Autodesk Inventor part; units mm, degrees
ref_plane "YZ Plane" through (0, 0, 0) normal (1, 0, 0) x (0, 1, 0)
ref_plane "XZ Plane" through (0, 0, 0) normal (0, 1, 0) x (-1, 0, 0)
ref_plane "XY Plane" through (0, 0, 0) normal (0, 0, 1) x (1, 0, 0)
sketch "Sketch1" plane through (0, 0, 0) normal (0, 1, 0) x (-1, 0, 0)
  line L0 (-175, 200) -> (175, 200)
  line L1 (175, 200) -> (175, -200)
  line L2 (175, -200) -> (-175, -200)
  line L3 (-175, -200) -> (-175, 200)
  line L4 (-175, 200) -> (175, -200) construction
  line L5 (175, 200) -> (-175, -200) construction
  point P0 (0, 0)
  point P1 (0, 0)
  dimension "d0" = 350
  dimension "d1" = 400
extrude "Extrusion1" add sketch "Sketch1" along normal blind 2
sketch "Sketch2" plane through (0, 0, 0) normal (0, -1, 0) x (1, 0, 0)
  line L0 (175, 200) -> (175, -200) construction
  line L1 (-175, 200) -> (175, 200) construction
  line L2 (175, 155) -> (125, 155)
  line L3 (125, 155) -> (125, 135)
  line L4 (125, 135) -> (175, 135)
  line L5 (175, 135) -> (175, 155)
  line L6 (0, 0) -> (119.5058, 0) construction
  line L7 (175, -155) -> (125, -155)
  line L8 (125, -155) -> (125, -135)
  line L9 (125, -135) -> (175, -135)
  line L10 (175, -135) -> (175, -155)
  line L11 (175, -200) -> (-175, -200) construction
  line L12 (0, 0) -> (0, 102.1582) construction
  line L13 (-175, 155) -> (-125, 155)
  line L14 (-125, 155) -> (-125, 135)
  line L15 (-125, 135) -> (-175, 135)
  line L16 (-175, 135) -> (-175, 155)
  line L17 (-175, -155) -> (-125, -155)
  line L18 (-125, -155) -> (-125, -135)
  line L19 (-125, -135) -> (-175, -135)
  line L20 (-175, -135) -> (-175, -155)
  line L21 (125, 135) -> (145, 135)
  line L22 (145, 135) -> (145, 200)
  line L23 (145, 200) -> (125, 200)
  line L24 (125, 200) -> (125, 135)
  line L25 (125, -135) -> (145, -135)
  line L26 (145, -135) -> (145, -200)
  line L27 (145, -200) -> (125, -200)
  line L28 (125, -200) -> (125, -135)
  point P0 (150, 155)
  point P1 (150, -155)
  point P2 (-150, 155)
  point P3 (-150, -155)
  dimension "d4" = 50
  dimension "d5" = 20
  dimension "d6" = 45
  dimension "d9" = 20
  dimension "d10" = 20
extrude "Extrusion2" add sketch "Sketch2" along normal blind 2 contours L22 L4 L3 L2 | L2 L24 L23 L22 | L26 L27 L28 L7 | L7 L8 L9 L26 | L13 L14 L15 L16 | L20 L19 L18 L17
sketch "Sketch3" plane through (145, 0, 200) normal (1, 0, 0) x (0, 0, -1)
  line L0 (400, 2) -> (0, 2) construction
  line L1 (0, 2) -> (-20, 2)
  line L2 (0, -2) -> (-20, -2)
  line L3 (-20, -2) -> (-20, 2)
  arc A0 (-20, -2) -> (-20, -37) centre (-20, -19.5) ccw
  line L4 (-20, -2) -> (-20, -37) construction
  line L5 (-20, -2) -> (15, -2) construction
  arc A1 (-20, 2) -> (-20, -41) centre (-20, -19.5) ccw
  line L6 (-20, 2) -> (-20, -44.4597)
  line L7 (0, 2) -> (0, -2)
  point P0 (200, 0)
  point P1 (-20, -41)
  point P2 (-20, -37)
  dimension "d11" = 20
  dimension "d12" = 35
  dimension "d13" = 90
  dimension "d14" = 4
extrude "Extrusion3" add sketch "Sketch3" against normal up to surface (20 mm away) contours L7 L2 L3 L1 | L3 A0 L6 A1
mirror "Mirror1" about plane through (0, 0, 0) normal (0, 0, 1) of "Extrusion3"
sketch "Sketch4" plane through (-175, 0, 155) normal (0, 0, 1) x (1, 0, 0)
  line L0 (139.9111, 57.1289) -> (-260.0889, 57.1289) construction
  line L1 (0, 1.8433) -> (-35, 1.8433)
  line L2 (0, -2) -> (-35, -2)
  line L3 (-35, -2) -> (-35, 1.8433)
  arc A0 (-35, -2) -> (-35, -37) centre (-35, -19.5) ccw
  line L4 (-35, -2) -> (-35, -37) construction
  line L5 (-280.0889, 53.1289) -> (-245.0889, 53.1289) construction
  arc A1 (-35, 1.8433) -> (-35, -41) centre (-35, -19.5784) ccw
  line L6 (-35, 1.8433) -> (-35, -44.4597)
  line L7 (0, 1.8433) -> (0, -2)
  point P0 (175, 0)
  point P1 (-60.0889, 55.1289)
  point P2 (-280.0889, 14.1289)
  point P3 (-280.0889, 18.1289)
  point P4 (-35, -37)
  point P5 (-35, -2)
  point P6 (-35, -2)
  dimension "d17" = 35
  dimension "d18" = 35
  dimension "d19" = 90
  dimension "d20" = 4
extrude "Extrusion4" add sketch "Sketch4" against normal up to surface (20 mm away) contours L7 L2 L3 L1 | L3 A0 L6 A1
mirror "Mirror2" about plane through (0, 0, 0) normal (0, 0, 1) of "Extrusion4"
Input: part model. Units: mm. Frame: model coordinates. A direction names the side the tool comes from. Coordinates: 2 decimals unless noted, no trailing zeros. Write each loop counter-clockwise with the first axis right and the second up, starting at its lowest first coordinate (ties: lowest second). Pieces come first, ordered by that corner, then holes. Notation, with made-up numbers: M 44.25,-33.5 L 75.25,-33.5 A22 ccw 75.25,-14.5 Z; hole C 21.5,84.25 d11. An arc over 180 degrees is marked long. Answer as a JSON object with one key per item and string values. Group by question number.
(1) Section D-D on x = -25.5. Output: boundary loops of the cut face in (y, z).
(2) Section C-C on z = -95. Output: boundary loops of the cut face in (x, y), plus the area to 3 significant figures.
(3) Mould query, pull axis Y, two halves, no side actions, for faces 1 (the face through (-227.496, -19.115, 145.14)), 2 (the face through (2, 2, 3)), 3 (the face through (-202, 0, -155)). Classes: pulls with the +Y half, pulls with the -Y half, needs draft (parallel to the pull), parting line crosses it, or undercut.
(4) Ray query, line 1 along Y through (x, z) = (11, 20); line 2 along Z through (x, y) = (137, -11); line 3 along X through (y, z) = (-31.5, 144). Return the intervals inside material, ascending. Write a range as [from, to].
(5) Section A-A on x = -154. Output: boundary loops of the cut face in (y, z), plus the area to 3 significant figures.
(6) Contact query for flat-ended pins moving along their axis: P1, Ø1, axis at x = 152.5, y = 1, coming from the -Z side; P2, Ø2, axis at y = 1, z = 73, coming from the -X side; P3, Ø1, axis at y = -1, z = 141, coming from the +X side; P4, Ø21.5, axis at x = -176, y = -21.5, coming from the +Z side. Output: stop coordinate, or through.
(7) Set-up query: faces 4 (the face through (-202, 0, 135)), 5 (the face through (-227.496, -19.885, -145.14)), 6 (the face through (135, -2, 177)). Return all of +Z, -Z, +X, -X, +Y, -Y with unobstructed straight access to the full face (end or side cutting, diameter ignored); none if empty.
(8) Section B-B on y = -19.5. Output: boundary loops of the cut face in (x, z), plus the area to 3 significant figures.
Result set:
{
 "1": {"outline": "M 0,-200 L 2,-200 L 2,200 L 0,200 Z"},
 "2": {"outline": "M -175,0 L 175,0 L 175,2 L -175,2 Z", "area": "700 mm2"},
 "3": {"face 1": "undercut", "face 2": "pulls with the +Y half", "face 3": "needs draft"},
 "4": {"line 1": "y = [0, 2]", "line 2": "z = [-239.75, -235.3], [235.3, 239.75]", "line 3": "x = [-227.8, -222.74]"},
 "5": {"outline": "M -2,-155 L 0,-155 L 0,-200 L 2,-200 L 2,200 L 0,200 L 0,155 L -2,155 L -2,135 L 0,135 L 0,-135 L -2,-135 Z", "area": "880 mm2"},
 "6": {"P1": "stops at z = -200", "P2": "stops at x = -175", "P3": "stops at x = 145", "P4": "passes through"},
 "7": {"face 4": "-X, -Y", "face 5": "+Z, -Z, +X", "face 6": "+X, -Y"},
 "8": {"outline": "M -231.42,-155 L -227.5,-155 L -227.5,-135 L -231.42,-135 Z; M -231.42,135 L -227.5,135 L -227.5,155 L -231.42,155 Z; M 125,-241.5 L 145,-241.5 L 145,-237.5 L 125,-237.5 Z; M 125,237.5 L 145,237.5 L 145,241.5 L 125,241.5 Z", "area": "317 mm2"}
}
